Can you work these out from the model? Positions are in its coordinate system, mm. A direction names the side the tool comes from. Round coordinates to 2 decimals unless told otherwise and drop trailing zeros. Order: outer loops, then holes, each group sorted by start corner. A loop starts at its lowest first (then second) coordinate and runs counter-clockwise, first axis right, second up. Notation, with made-up numbers: M 76.25,-40 L 85.25,-40 A22 cw 85.25,-32 Z; hole C 33.5,43.5 d8. An arc over 180 degrees is marked long. Answer as a JSON object with one key per item and string values. Group by question number.
Autodesk Inventor part; units mm, degrees
ref_plane "YZ Plane" through (0, 0, 0) normal (1, 0, 0) x (0, 1, 0)
ref_plane "XZ Plane" through (0, 0, 0) normal (0, 1, 0) x (-1, 0, 0)
ref_plane "XY Plane" through (0, 0, 0) normal (0, 0, 1) x (1, 0, 0)
sketch "Sketch1" plane through (0, 0, 0) normal (0, 0, 1) x (1, 0, 0)
  line L0 (-5.3333, 0.9286) -> (39.6667, 0.9286)
  line L1 (39.6667, 0.9286) -> (39.6667, -1.0714)
  line L2 (39.6667, -1.0714) -> (-5.3333, -1.0714)
  line L3 (-5.3333, -1.0714) -> (-5.3333, 0.9286)
  line L4 (-5.3333, 18.9286) -> (38.4017, 18.9286)
  line L5 (38.4017, 18.9286) -> (38.4017, 16.9286)
  line L6 (38.4017, 16.9286) -> (-5.3333, 16.9286)
  line L7 (-5.3333, 16.9286) -> (-5.3333, 18.9286)
  line L8 (16.5342, 16.9286) -> (15.5342, 16.9286)
  line L9 (15.5342, 16.9286) -> (15.5342, 0.9286)
  line L10 (15.5342, 0.9286) -> (16.5342, 0.9286)
  line L11 (16.5342, 0.9286) -> (16.5342, 16.9286)
  line L12 (16.5342, 16.9286) -> (17.5342, 16.9286)
  line L13 (17.5342, 16.9286) -> (17.5342, 0.9286)
  line L14 (17.5342, 0.9286) -> (16.5342, 0.9286)
  line L15 (16.5342, 0.9286) -> (16.5342, 16.9286)
  point P0 (0, 0)
  dimension "d0" = 2
  dimension "d1" = 45
  dimension "d2" = 2
  dimension "d3" = 1
  dimension "d4" = 1
  dimension "d5" = 20
extrude "Extrusion1" add sketch "Sketch1" along normal blind 10
sketch "Sketch2" plane through (-5.3333, 18.9286, 0) normal (0, 1, 0) x (1, 0, 0)
  circle A0 centre (10, -5) radius 3
  circle A1 centre (35, -5) radius 3
  line L0 (0, 0) -> (0, -10)
  line L1 (45, 0) -> (45, -10)
  line L2 (43.735, 0) -> (0, 0)
  point P0 (5.3333, 0)
  dimension "d8" = 6
  dimension "d9" = 6
  dimension "d10" = 10
  dimension "d11" = 10
  dimension "d12" = 5
  dimension "d13" = 5
extrude "Extrusion2" cut sketch "Sketch2" against normal blind 20
fillet "Fillet1" radius 2 4 edges at (17.5342, 0.9286, 5) (15.5342, 0.9286, 5) (17.5342, 16.9286, 5) (15.5342, 16.9286, 5)
properties part number "Slider ver2"
Item 1: Suppose I cut it at C-C, the plane z = 8.5. Write out the boundary of the cut face in (x, y), and give its area (3 significant figures).
Item 2: On a 3-axis mill with a long thin cutter (end or side, diameter ignored), from which of +Z, -Z, +X, -X, +Y, -Y can I reach the whole of each face in a straight line? I mean faces 1 (the face through (16, 18.929, 5)), 2 (the face through (27, 16.929, 3)), 3 (the face through (38.402, 18, 5)), 4 (the face through (2, 16.929, 3)). Say none if no direction works.
Item 3: I'm going to push flat-ended pins straight in: pin 1 Ø3 at (y, z) = (11.5, 3) entering from +X; pin 2 Ø3.5 at (x, z) = (4.67, 5) entering from +Y; pin 3 Ø3 at (y, z) = (7.5, 4) entering from -X; pin 4 Ø2 at (y, z) = (17.5, 3.5) entering from +X. Where does each tip first touch, or does it pass through?
Item 4: Suppose I cut it at B-B, the plane x = 9.5. Write out the boundary of the cut face in (y, z).
Item 5: If we mould it in two halves opening along Z, with no side actions, what happens to faces 5 (the face through (17, 9, 10)), 6 (the face through (-5.333, 18, 5)), 7 (the face through (17, 9, 0)), 8 (the face through (29.276, 17.943, 2.026))? For each: +Z half, -Z half, draft (parallel to the pull), parting line (faces both ways), or undercut.
Item 6: Suppose I cut it at D-D, the plane y = 12. Write out the boundary of the cut face in (x, z), and give its area (3 significant figures).
Item 7: Suppose I cut it at A-A, the plane z = 5. State how many separate pieces and enclosed holes the cut face has, and give its area (3 significant figures).
Item 8: I need wall thicknesses on line 1 (X direction, y = -0.3, z = 5); line 2 (X direction, y = 18.5, z = 5); line 3 (Y direction, x = 27.5, z = 9.75). Which ranges of each line are inside material? Lowest first, please.
Computed:
{
 "1": {"outline": "M -5.33,-1.07 L 39.67,-1.07 L 39.67,0.93 L 19.53,0.93 A2 cw 17.53,2.93 L 17.53,14.93 A2 cw 19.53,16.93 L 38.4,16.93 L 38.4,18.93 L -5.33,18.93 L -5.33,16.93 L 13.53,16.93 A2 cw 15.53,14.93 L 15.53,2.93 A2 cw 13.53,0.93 L -5.33,0.93 Z", "area": "213 mm^2"},
 "2": {"face 1": "+Z, -Z, +X, -X, +Y", "face 2": "+Z, -Z, +X", "face 3": "+Z, -Z, +X, +Y", "face 4": "+Z, -Z, -X"},
 "3": {"pin 1": "stops at x = 17.53", "pin 2": "passes through", "pin 3": "stops at x = 15.53", "pin 4": "stops at x = 38.4"},
 "4": {"outline": "M -1.07,0 L 0.93,0 L 0.93,10 L -1.07,10 Z; M 16.93,0 L 18.93,0 L 18.93,10 L 16.93,10 Z"},
 "5": {"face 5": "+Z half", "face 6": "draft", "face 7": "-Z half", "face 8": "undercut"},
 "6": {"outline": "M 15.53,0 L 17.53,0 L 17.53,10 L 15.53,10 Z", "area": "20.0 mm^2"},
 "7": {"separate pieces": "5", "enclosed holes": "0", "area": "165 mm^2"},
 "8": {"line 1": "x = -5.33 to 1.67, 7.67 to 26.67, 32.67 to 39.67", "line 2": "x = -5.33 to 1.67, 7.67 to 26.67, 32.67 to 38.4", "line 3": "y = -1.07 to 0.93, 16.93 to 18.93"}
}
